Build history of the part. All positions in model axes, mm. A direction names the side the tool comes from. Coordinates: 2 decimals unless noted, no trailing zeros. Loops run counter-clockwise (first coordinate to the right, second up) from the corner with the lowest first, then second, coordinate; pieces in that order, holes last. Notation, with made-up numbers: M 77.5,-18 L 123.5,-18 A20 cw 123.5,-4 Z; hole C 62,-16.5 d9. An arc over 180 degrees is marked long. Write each question's results on one line, items separated by ' | '. Start each with the question number.
from build123d import *

# Parameters (mm, degrees)
PAD003_DEPTH       = 1.2
PAD004_DEPTH       = 9.6
PAD005_DEPTH       = 1.2
PAD006_DEPTH       = 1
PAD007_DEPTH       = 1
CHAMFER001_1_SIZE2 = 0.8
CHAMFER001_1_SIZE  = 1
CHAMFER001_2_SIZE2 = 0.8
CHAMFER001_2_SIZE  = 1
FILLET001_R        = 1


with BuildPart() as part:
    # Sketch006 → Pad003 (new body)
    with BuildSketch(Plane.XY):
        with BuildLine():
            ThreePointArc((-94.2875364362, 7.682478298), (-94.6, 0), (-94.2875364362, -7.682478298))
            Line((-94.2875364362, -7.682478298), (-82.6504571335, -7.682478298))
            Line((-82.6504571335, 7.682478298), (-82.6504571335, -7.682478298))
            Line((-94.2875364362, 7.682478298), (-82.6504571335, 7.682478298))
        make_face()
    extrude(amount=PAD003_DEPTH)

    # Sketch007 → Pad004 (join)
    with BuildSketch(Plane.XY.offset(1.2)):
        with BuildLine():
            ThreePointArc((-94.2875364362, 7.682478298), (-94.6, 0), (-94.2875364362, -7.682478298))
            Line((-93.0835083525, -7.682478298), (-94.2875364362, -7.682478298))
            ThreePointArc((-93.0835083525, 7.682478298), (-93.4, 0), (-93.0835083525, -7.682478298))
            Line((-94.2875364362, 7.682478298), (-93.0835083525, 7.682478298))
        make_face()
    extrude(amount=PAD004_DEPTH)

    # Sketch008 → Pad005 (join)
    with BuildSketch(Plane.XY.offset(10.8)):
        with BuildLine():
            ThreePointArc((-94.2875364362, 7.682478298), (-94.6, 0), (-94.2875364362, -7.682478298))
            Line((-94.2875364362, -7.682478298), (-82.6504571335, -7.682478298))
            Line((-82.6504571335, 7.682478298), (-82.6504571335, -7.682478298))
            Line((-94.2875364362, 7.682478298), (-82.6504571335, 7.682478298))
        make_face()
    extrude(amount=PAD005_DEPTH)

    # Sketch009 → Pad006 (join)
    with BuildSketch(Plane.XY.offset(1.2)):
        with BuildLine():
            ThreePointArc((-84.2504571335, 7.682478298), (-84.6, 0), (-84.2504571335, -7.682478298))
            Line((-82.6504571335, -7.682478298), (-84.2504571335, -7.682478298))
            Line((-82.6504571335, 7.682478298), (-82.6504571335, -7.682478298))
            Line((-84.2504571335, 7.682478298), (-82.6504571335, 7.682478298))
        make_face()
    extrude(amount=PAD006_DEPTH)

    # Sketch010 → Pad007 (join)
    with BuildSketch(Plane.XY.offset(10.8)):
        with BuildLine():
            ThreePointArc((-84.2504571335, 7.682478298), (-84.6, 0), (-84.2504571335, -7.682478298))
            Line((-82.6504571335, -7.682478298), (-84.2504571335, -7.682478298))
            Line((-82.6504571335, 7.682478298), (-82.6504571335, -7.682478298))
            Line((-84.2504571335, 7.682478298), (-82.6504571335, 7.682478298))
        make_face()
    extrude(amount=-PAD007_DEPTH)

    # Chamfer001 1
    chamfer001_1_edges = [part.edges().sort_by_distance(p)[0] for p in [
        (-82.650457, 0, 2.2),
    ]]
    chamfer001_1_side = part.faces().sort_by_distance((-83.56998, 0, 2.2))[0]
    chamfer(chamfer001_1_edges, length=CHAMFER001_1_SIZE, length2=CHAMFER001_1_SIZE2, reference=chamfer001_1_side)

    # Chamfer001 2
    chamfer001_2_edges = [part.edges().sort_by_distance(p)[0] for p in [
        (-82.650457, 0, 9.8),
    ]]
    chamfer001_2_side = part.faces().sort_by_distance((-83.56998, 0, 9.8))[0]
    chamfer(chamfer001_2_edges, length=CHAMFER001_2_SIZE, length2=CHAMFER001_2_SIZE2, reference=chamfer001_2_side)

    # Fillet001
    fillet001_edges = [part.edges().sort_by_distance(p)[0] for p in [
        (-94.6, 0, 0),
        (-94.6, 0, 12),
        (-82.650457, 0, 0),
        (-82.650457, 0, 12),
        (-83.950457, -7.682478, 9.8),
        (-83.950457, -7.682478, 2.2),
        (-83.950457, 7.682478, 2.2),
        (-83.950457, 7.682478, 9.8),
    ]]
    fillet(fillet001_edges, radius=FILLET001_R)


solid = part.part
1. Pin check, flat tips, straight feed: pin 1 (1 mm diameter, centred on x = -89.5, z = 3, fed in from -Y); pin 2 (3 mm diameter, centred on x = -84.5, z = 3.5, fed in from +Y). Stop position of each tip, or through.
2. Which spindle directions (+Z, -Z, +X, -X, +Y, -Y) get a long thin tool onto all of the face, cutting with end or side? Do faces 1 (the cylindrical face through (-83.692, -7.495, 10.217)), 2 (the cylindrical face through (-83.67, 7.51, 1.76)), 3 (the flat face through (-83.14, 0.11, 1.79)), 4 (the cylindrical face through (-93.4, 0.1, 5.9)). Say none if no direction does.
3. Mould opens along X. For faces 5 (the flat face through (-83.14, 0.11, 10.21)), 6 (the flat face through (-89, 0, 10.8)), 7 (the flat face through (-94, -7.682, 6)) say: +X half, -X half, draft (parallel to the pull), parting line (faces both ways), or undercut.
4. Band-saw the part on B-B, the plane z = 3.5. List the corners of the cut face in (x, y), plus the area to 3 significant figures.
5. Band-saw the part on A-A, the plane x = -86.25. List the corners of the cut face in (y, z).
6. Wall check: line 1 along Z through (x, y) = (-87.5, -4.25); line 2 along Z through (x, y) = (-83.75, -0.75); line 3 along X through (y, z) = (-0.5, 5.5). Give the ranges that are in metal, low to high.
Checked values:
1) pin 1: through | pin 2: y = 7.26
2) face 1: +X, -Y | face 2: +X, +Y | face 3: +X, +Y, -Y | face 4: none
3) face 5: +X half | face 6: undercut | face 7: draft
4) outline: M -94.29,-7.68 L -93.08,-7.68 A93.4 cw -93.08,7.68 L -94.29,7.68 A94.6 ccw Z | area: 18.5 mm²
5) outline: M -7.68,0 L 7.68,0 L 7.68,1.2 L -7.68,1.2 Z; M -7.68,10.8 L 7.68,10.8 L 7.68,12 L -7.68,12 Z
6) line 1: 0 to 1.2, 10.8 to 12 | line 2: 0 to 2.2, 9.8 to 12 | line 3: -94.6 to -93.4
